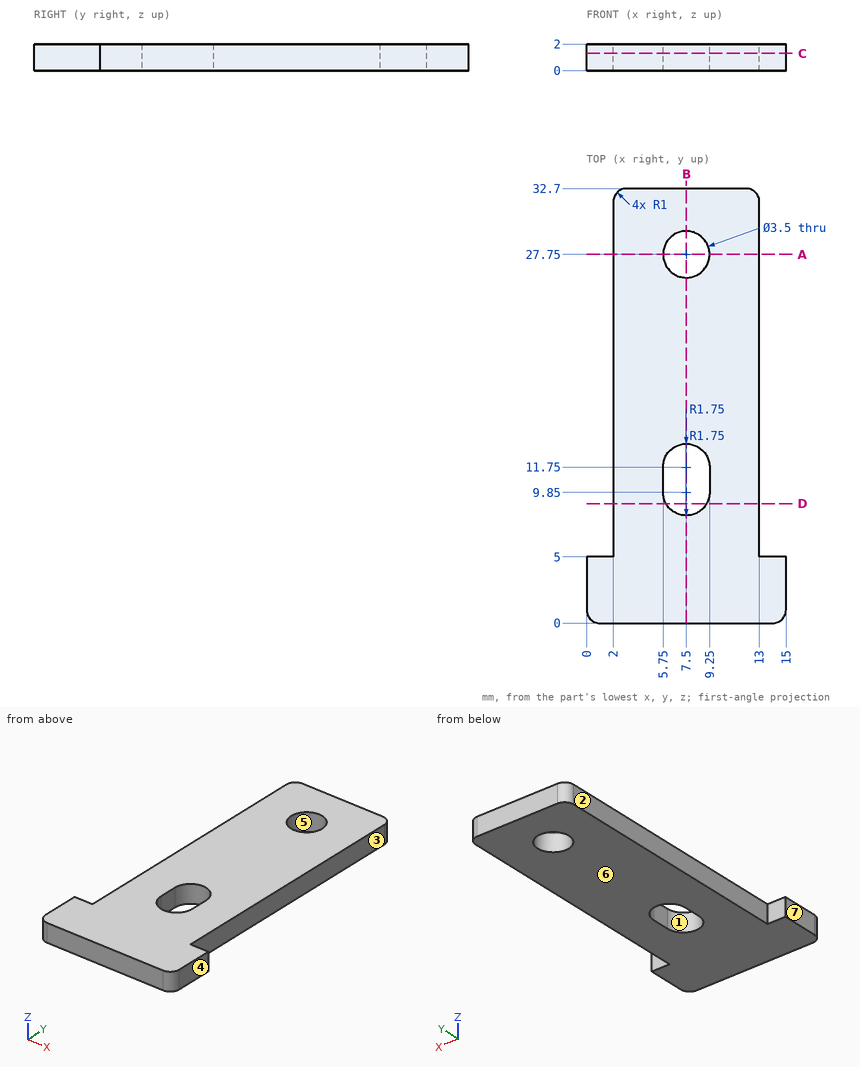
Here's the drawing with two shaded views (mm, measured from the low corner). I have some questions. A direction names the side the tool comes from. Coordinates: 2 decimals unless noted, no trailing zeros. Loops run counter-clockwise (first coordinate to the right, second up) from the corner with the lowest first, then second, coordinate; pieces in that order, holes last. Notation, with made-up numbers: (86.25, 7.25) -> (139.25, 7.25) arc R14 ccw to (139.25, 18.25) -> close; hole circle Ø2 at (18.5, 64.25). An arc over 180 degrees is marked (long way). Use one line per item in the form item = value. Start each with the question number.
(1) If we section it at C-C (z = 1.3): Please give me the cut outline in (x, y), then the cut area to 3 significant figures.
(2) Please list where these lines run through material, in increasing order: line 1 along Y through (x, z) = (7.5, 0.7); line 2 along X through (y, z) = (10, 1.6); line 3 along X through (y, z) = (21, 1.65).
(3) If we section it at A-A (y = 27.75): Please give me the cut outline in (x, z), then the cut area to 3 significant figures.
(4) Will this pin go through, and if not, where does the flat tip stop? pin 1 (1 mm diameter, centred on y = 20, z = 0.5, fed in from -X).
(5) On a 3-axis mill with a long thin cutter (end or side, diameter ignored), from which of +Z, -Z, +X, -X, +Y, -Y can I reach the whole of each face in a straight line? I mean the marked faces 1, 2 and 3. Say none if no direction works.
(6) If we section it at B-B (x = 7.5): Please give me the cut outline in (y, z).
(7) We'd pull the mould along X, two halves only. Please class the marked faces 4, 5, 6 and 7: pulls with the +X half, pulls with the -X half, needs draft (parallel to the pull), parting line crosses it, or undercut.
(8) If we section it at D-D (y = 9): Please give me the cut outline in (x, z), then the cut area to 3 significant figures.
Verdict:
q1.outline = (0, 1) arc R1 ccw to (1, 0) -> (14, 0) arc R1 ccw to (15, 1) -> (15, 5) -> (13, 5) -> (13, 31.7) arc R1 ccw to (12, 32.7) -> (3, 32.7) arc R1 ccw to (2, 31.7) -> (2, 5) -> (0, 5) -> close; hole (5.75, 9.85) arc R1.75 ccw to (9.25, 9.85) -> (9.25, 11.75) arc R1.75 ccw to (5.75, 11.75) -> close; hole circle Ø3.5 at (7.5, 27.75)
q1.area = 353 mm²
q2.line_1 = 0 to 8.1, 13.5 to 26, 29.5 to 32.7
q2.line_2 = 2 to 5.75, 9.25 to 13
q2.line_3 = 2 to 13
q3.outline = (2, 0) -> (5.75, 0) -> (5.75, 2) -> (2, 2) -> close; (9.25, 0) -> (13, 0) -> (13, 2) -> (9.25, 2) -> close
q3.area = 15.0 mm²
q4.pin_1 = 2
q5.face_1 = +Z, -Z
q5.face_2 = +Z, -Z, -X, +Y
q5.face_3 = +Z, -Z, +X, +Y
q6.outline = (0, 0) -> (8.1, 0) -> (8.1, 2) -> (0, 2) -> close; (13.5, 0) -> (26, 0) -> (26, 2) -> (13.5, 2) -> close; (29.5, 0) -> (32.7, 0) -> (32.7, 2) -> (29.5, 2) -> close
q7.face_4 = pulls with the +X half
q7.face_5 = undercut
q7.face_6 = needs draft
q7.face_7 = pulls with the -X half
q8.outline = (2, 0) -> (5.97, 0) -> (5.97, 2) -> (2, 2) -> close; (9.03, 0) -> (13, 0) -> (13, 2) -> (9.03, 2) -> close
q8.area = 15.9 mm²
